from build123d import *

# Parameters (mm, degrees)
REVOLVE3_ANGLE = 270


with BuildPart() as part:
    # Sketch1 → Revolve3 (revolve)
    with BuildSketch(Plane(origin=(0, 0, 0), x_dir=(0, 0, -1), z_dir=(1, 0, 0))):
        with BuildLine():
            add(Edge.make_bspline(
                [(115.7465953, -1.008655183), (114.892603244, -1.634204905), (114.264623631, -1.959063002), (113.639238781, 0)],
                knots=[0.465469081, 0.465469081, 0.465469081, 0.465469081, 1, 1, 1, 1], degree=3))
            add(Edge.make_bspline(
                [(113.639238781, 0), (113.639238781, 12.165321536), (68.639238781, 18.568122345)],
                knots=[3.141592654, 3.141592654, 3.141592654, 4.158127146, 4.158127146, 4.158127146], degree=2, weights=[1, 0.873589088, 1]))
            Line((68.639238781, 18.568122345), (68.639238781, 13.568122345))
            Line((68.639238781, 13.568122345), (63.639238781, 13.568122345))
            Line((63.639238781, 13.568122345), (63.639238781, 19.232101882))
            add(Edge.make_bspline(
                [(63.639238781, 19.232101882), (18.639238781, 24.801791276), (-26.360761219, 19.232101882)],
                knots=[1.077097687, 1.077097687, 1.077097687, 2.064494967, 2.064494967, 2.064494967], degree=2, weights=[1, 0.880586152, 1]))
            Line((-26.360761219, 19.232101882), (-26.360761219, 13.568122345))
            Line((-26.360761219, 13.568122345), (-31.360761219, 13.568122345))
            Line((-31.360761219, 13.568122345), (-31.360761219, 18.568122345))
            add(Edge.make_bspline(
                [(-31.360761219, 18.568122345), (-64.825670935, 13.806585656), (-73.837058596, 5)],
                knots=[2.125058161, 2.125058161, 2.125058161, 2.910578584, 2.910578584, 2.910578584], degree=2, weights=[1, 0.923856138, 1]))
            Line((-73.837058596, 5), (-79.893391232, 5))
            add(Edge.make_bspline(
                [(118.639238781, 0), (118.639238781, 26.883956752), (27.204780174, 29.186713196), (-64.229678433, 31.489469639), (-79.893391232, 5)],
                knots=[0, 0, 0, 1.485035825, 1.485035825, 2.970071651, 2.970071651, 2.970071651], degree=2, weights=[1, 0.736768422, 1, 0.736768422, 1]))
            add(Edge.make_bspline(
                [(118.639238781, 0), (117.988045153, -1.021098807), (117.023830916, -1.357317272), (115.7465953, -1.008655183)],
                knots=[0, 0, 0, 0, 0.670728869, 0.670728869, 0.670728869, 0.670728869], degree=3))
        make_face()
    revolve(axis=Axis((0, -10.77, -129.717244309), (0, 0, 1)), revolution_arc=REVOLVE3_ANGLE)


solid = part.part
Model file for the job. Use its own axes, mm. A direction names the side the tool comes from. Round coordinates to 2 decimals unless told otherwise and drop trailing zeros. Write each question's results on one line, items separated by ' | '.
(1) Pin check, flat tips, straight feed: pin 1 (24.5 mm diameter, centred on x = 30.5, z = -9.5, fed in from +Y); pin 2 (10 mm diameter, centred on x = -0.5, y = -17, fed in from -Z); pin 3 (9 mm diameter, centred on y = 8, z = -8.5, fed in from +X); pin 4 (10 mm diameter, centred on x = 4.5, z = 49, fed in from -Y). Stop position of each tip, or through.
Answer below:
pin 1: stops at y = -10.77 | pin 2: stops at z = -118.64 | pin 3: stops at x = -22.66 | pin 4: stops at y = -44.19
(2) Wall check: L1, parallel to Y at x = -4, z = 57.5; L2, parallel to X at y = -19, z = -44; L3, parallel to X at y = -21.5, z = 46. Give the ranges that are in metal, low to high.
Answer below:
L1: y = -40.26 to -34.26, 12.72 to 18.72 | L2: x = -38.23 to -30.73, 30.73 to 38.23 | L3: x = -31.34 to -24.53, 24.53 to 31.34
(3) Mould opens along Y. For faces 1 (the flat face through (33, -10.77, -27)), 2 (the flat face through (0, 22, -27)), 3 (the flat face through (-18, -29, 26.361)) say: released by +Y, released by -Y, zero draft, split by the parting line, or undercut.
Answer below:
face 1: released by +Y | face 2: zero draft | face 3: undercut
(4) 3-axis set-ups, long thin cutter, end or side, ignore diameter. For faces 4 (the flat face through (-18, -28, 31.361)), 5 (the cylindrical face through (-11.51, -21.55, 76.91)): which of +Z, -Z, +X, -X, +Y, -Y reach the whole face in a straight line?
Answer below:
face 4: none | face 5: +Z
